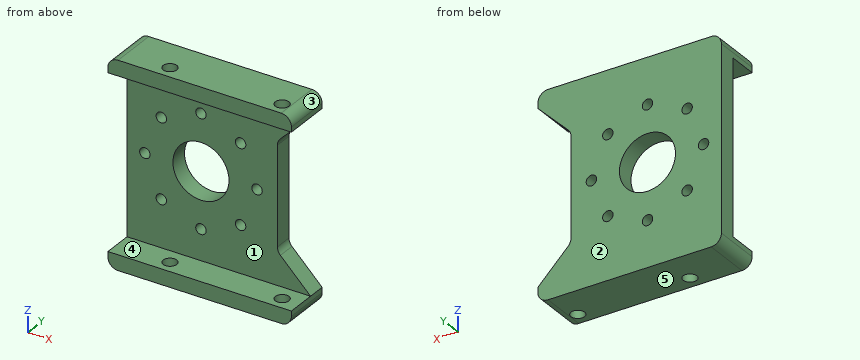
Autodesk Inventor part; units mm, degrees
ref_plane "YZ Plane" through (0, 0, 0) normal (1, 0, 0) x (0, 1, 0)
ref_plane "XZ Plane" through (0, 0, 0) normal (0, 1, 0) x (-1, 0, 0)
ref_plane "XY Plane" through (0, 0, 0) normal (0, 0, 1) x (1, 0, 0)
sketch "Sketch2" plane through (0, 0, 0) normal (0, 1, 0) x (-1, 0, 0)
  line L0 (18, 20) -> (-18, 20)
  line L1 (-18, 20) -> (-18, -20)
  line L2 (-18, -20) -> (18, -20)
  line L3 (18, -20) -> (18, 20)
  line L4 (18, 20) -> (-18, -20) construction
  line L5 (-18, 20) -> (18, -20) construction
  point P0 (0, 0)
  dimension "d0" = 36
  dimension "d1" = 40
extrude "Extrusion1" add sketch "Sketch2" along normal blind 9.3
sketch "Sketch3" plane through (0, 0, 0) normal (0, -1, 0) x (1, 0, 0)
  line L0 (-18, -17) -> (18, -17)
  line L1 (18, -17) -> (18, 17)
  line L2 (18, 17) -> (-18, 17)
  line L3 (-18, 17) -> (-18, -17)
  line L4 (-18, -17) -> (18, 17) construction
  line L5 (18, -17) -> (-18, 17) construction
  point P0 (0, 0)
  dimension "d4" = 36
  dimension "d5" = 34
extrude "Extrusion2" cut sketch "Sketch3" against normal blind 5.8
sketch "Sketch4" plane through (18, 0, -20) normal (0, 0, -1) x (-1, 0, 0)
  line L0 (0, 0) -> (36, 0)
  line L1 (36, 0) -> (36, 9.3)
  line L2 (0, 9.3) -> (36, 9.3)
  line L3 (0, 0) -> (0, 9.3)
  line L4 (36, 0) -> (0, 0) construction
  line L5 (0, 0) -> (0, 2.6) construction
  line L6 (0, 0) -> (0, 9.3) construction
  line L7 (0, 2.6) -> (3.5, 2.6) construction
  line L8 (3.5, 2.6) -> (25.5, 2.6) construction
  circle A0 centre (3.5, 2.6) radius 1.35
  circle A1 centre (25.5, 2.6) radius 1.35
  point P0 (18, 0)
  dimension "d8" = 2.6
  dimension "d9" = 3.5
  dimension "d10" = 22
  dimension "d11" = 180
  dimension "d12" = 2.7
  dimension "d13" = 2.7
extrude "Extrusion3" cut sketch "Sketch4" against normal up to surface (40 mm away) contours A0 | A1
sketch "Sketch5" plane through (0, 9.3, 0) normal (0, 1, 0) x (1, 0, 0)
  line L0 (18, -17) -> (18, 17)
  line L1 (18, 0) -> (7.5, 0)
  line L2 (18, 0) -> (28.5, 0) construction
  line L3 (7.5, 0) -> (-3.5, 0)
  line L4 (7.5, 0) -> (18.5, 0) construction
  circle A0 centre (7.5, 0) radius 1.025
  circle A1 centre (4.2782, 7.7782) radius 1.025
  circle A2 centre (-3.5, 11) radius 1.025
  circle A3 centre (-11.2782, 7.7782) radius 1.025
  circle A4 centre (-14.5, 0) radius 1.025
  circle A5 centre (-11.2782, -7.7782) radius 1.025
  circle A6 centre (-3.5, -11) radius 1.025
  circle A7 centre (4.2782, -7.7782) radius 1.025
  circle A8 centre (-3.5, 0) radius 5.5
  point P0 (0, 0)
  dimension "d16" = 10.5
  dimension "d17" = 180
  dimension "d18" = 11
  dimension "d19" = 180
  dimension "d20" = 2.05
  dimension "d23" = 360
  dimension "d25" = 11
extrude "Extrusion4" cut sketch "Sketch5" against normal up to surface (3.5 mm away)
sketch "Sketch6" plane through (0, 9.3, 0) normal (0, 1, 0) x (1, 0, 0)
  line L0 (18, 17) -> (-18, 17)
  line L1 (-18, 20) -> (-18, 17)
  line L2 (18, 20) -> (-18, 20)
  line L3 (18, 17) -> (18, 20)
  line L4 (-18, -17) -> (18, -17)
  line L5 (18, -20) -> (18, -17)
  line L6 (-18, -20) -> (18, -20)
  line L7 (-18, -17) -> (-18, -20)
  line L8 (18, -17) -> (18, 17)
  line L9 (18, 0) -> (11.5, 0)
  line L10 (11.5, 0) -> (11.5, 17)
  line L11 (11.5, 0) -> (11.5, -17)
  line L12 (18, 17) -> (11.5, 10.5)
  line L13 (18, 17) -> (27.1924, 17) construction
  line L14 (-18, -17) -> (18, -17)
  line L15 (18, -17) -> (11.5, -10.5)
  line L16 (18, -17) -> (27.1924, -17) construction
  point P0 (0, 0)
  dimension "d28" = 6.5
  dimension "d29" = 135
  dimension "d30" = 135
extrude "Extrusion5" cut sketch "Sketch6" against normal up to surface (3.5 mm away) contours L8 L9 L10 L12 | L8 L15 L11 L9
fillet "Fillet1" radius 2 6 edges at (11.5, 7.55, -10.5) (18, 4.65, -20) (11.5, 7.55, 10.5) (18, 4.65, 20) (-18, 4.65, 20) (-18, 4.65, -20)
properties part number "connector_shoulder_jasper"
Source: CAD feature listing. Evaluate the final solid. Frame: model axes, mm. Face numbers are marked on the shaded views. A direction names the side the tool comes from. Round coordinates to 2 decimals unless told otherwise and drop trailing zeros. Loops run counter-clockwise (first coordinate to the right, second up) from the corner with the lowest first, then second, coordinate; pieces in that order, holes last.
Q1. Section D-D, the plane y = 7.5. State how many separate pieces and enclosed holes the cut face has, plus the area to 3 significant figures.
Q2. Mould query, pull axis Z, two halves, no side actions, for the marked faces 1, 2 and 3. Classes: pulls with the +Z half, pulls with the -Z half, needs draft (parallel to the pull), parting line crosses it, or undercut.
Q3. Ray query, line 1 (Z direction, x = -3.5, y = 8.1) (3 decimals); line 2 (Z direction, x = 8, y = 1.25); line 3 (Y direction, x = 14.5, z = 18.15). Return the intervals inside material, ascending.
Q4. First-contact query: P1, Ø2.5, axis at x = -11.28, z = 7.78, coming from the -Y side; P2, Ø4, axis at y = 8.5, z = -2.5, coming from the +X side. Flat tips, straight axial feed; report the tip coordinate or a pass-through.
Q5. Section A-A, the plane z = 0. Return loops of the section in (x, y) (3 decimals).
Q6. Section B-B, the plane x = 14.5. Return loops of the section in (y, z), plus the area to 3 significant figures.
Q7. Section C-C, the plane x = -14.5. Return loops of the section in (y, z) (3 decimals).
Q8. Access query for the marked faces 4 and 5. Directions: +Z, -Z, +X, -X, +Y, -Y. A direction counts if a zero-diameter tool reaches every point of the face in a straight line with its end or side. Return the directions, or none.
Solutions:
1. separate pieces: 1
1. enclosed holes: 9
1. area: 1,140 mm2
2. face 1: undercut
2. face 2: needs draft
2. face 3: pulls with the +Z half
3. line 1: z = -20 to -12.025, -9.975 to -5.5, 5.5 to 9.975, 12.025 to 20
3. line 2: z = -20 to -17, 17 to 20
3. line 3: y = 0 to 1.25, 3.95 to 9.3
4. P1: stops at y = 5.8
4. P2: stops at x = 11.5
5. outline: (-18, 5.8) - (-15.525, 5.8) - (-15.525, 9.3) - (-18, 9.3) - close; (-13.475, 5.8) - (-9, 5.8) - (-9, 9.3) - (-13.475, 9.3) - close; (2, 5.8) - (6.475, 5.8) - (6.475, 9.3) - (2, 9.3) - close; (8.525, 5.8) - (11.5, 5.8) - (11.5, 9.3) - (8.525, 9.3) - close
6. outline: (0, -20) - (1.25, -20) - (1.25, -17) - (0, -17) - close; (0, 17) - (1.25, 17) - (1.25, 20) - (0, 20) - close; (3.95, -20) - (9.3, -20) - (9.3, -13.5) - (5.8, -13.5) - (5.8, -17) - (3.95, -17) - close; (3.95, 17) - (5.8, 17) - (5.8, 13.5) - (9.3, 13.5) - (9.3, 20) - (3.95, 20) - close
6. area: 64.1 mm2
7. outline: (0, -20) - (9.3, -20) - (9.3, -1.025) - (5.8, -1.025) - (5.8, -17) - (0, -17) - close; (0, 17) - (5.8, 17) - (5.8, 1.025) - (9.3, 1.025) - (9.3, 20) - (0, 20) - close
8. face 4: +X, -X, -Y
8. face 5: -Z, +X, -X, +Y, -Y
